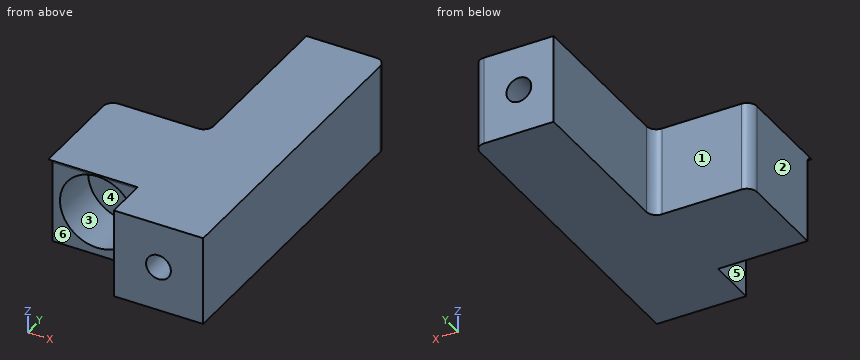
```python
from build123d import *

# Parameters (mm, degrees)
SKETCH1_W           = 9
SKETCH1_H           = 9
BOSS_EXTRUDE1_DEPTH = 15
SKETCH2_R           = 3.75
CUT_EXTRUDE1_DEPTH  = 5
SKETCH3_W           = 9
SKETCH3_H           = 9
BOSS_EXTRUDE2_DEPTH = 20
BOSS_EXTRUDE3_REACH = 25.859
SKETCH6_W           = 10
SKETCH6_H           = 9
CUT_EXTRUDE3_DEPTH  = 5
FILLET2_R           = 1
SKETCH7_W           = 8
SKETCH7_H           = 9
BOSS_EXTRUDE4_DEPTH = 12.5
SKETCH4_R           = 1.25
CUT_EXTRUDE2_DEPTH  = 36.478866949
FILLET3_R           = 1


with BuildPart() as part:
    # Sketch1 → Boss-Extrude1 (new body)
    with BuildSketch(Plane(origin=(0, 0, 0), x_dir=(1, 0, 0), z_dir=(0, 1, 0))):
        Rectangle(SKETCH1_W, SKETCH1_H)
    extrude(amount=BOSS_EXTRUDE1_DEPTH)

    # Sketch2 → Cut-Extrude1 (cut)
    with BuildSketch(Plane.XZ):
        with Locations(Location((0, 0, 0), (0, 0, 270))):
            Circle(SKETCH2_R)
    extrude(amount=-CUT_EXTRUDE1_DEPTH, mode=Mode.SUBTRACT)

    # Sketch3 → Boss-Extrude2 (add)
    with BuildSketch(Plane(origin=(0, 15, 0), x_dir=(1, 0, 0), z_dir=(0, 1, 0))):
        with Locations((9, 0)):
            Rectangle(SKETCH3_W, SKETCH3_H)
    extrude(amount=-BOSS_EXTRUDE2_DEPTH)

    # Boss-Extrude3: up to this face of the body (flat: up to its plane)
    boss_extrude3_end = Plane(part.part.faces().sort_by_distance((4.5, -2.5, 0))[0])
    # Sketch5 → Boss-Extrude3 (add, up to the picked face)
    with BuildSketch(Plane.ZY.offset(4.5), mode=Mode.PRIVATE) as boss_extrude3_sk1:
        with BuildLine():
            Line((4.5, -0.75), (4.5, 0))
            Line((4.5, 0), (3.75, 0))
            ThreePointArc((3.75, 0), (4.280330086, -0.219669914), (4.5, -0.75))
        make_face()
    boss_extrude3_tool1 = split(extrude(boss_extrude3_sk1.sketch, amount=-BOSS_EXTRUDE3_REACH, mode=Mode.PRIVATE), bisect_by=boss_extrude3_end, keep=Keep.BOTH, mode=Mode.PRIVATE)
    add(boss_extrude3_tool1.solids().sort_by(Axis((-4.5, -0.167526, 4.332474), (1, 0, 0)))[0])

    # Sketch6 → Cut-Extrude3 (cut)
    with BuildSketch(Plane(origin=(0, 15, 0), x_dir=(1, 0, 0), z_dir=(0, 1, 0))):
        with Locations((0.5, 0)):
            Rectangle(SKETCH6_W, SKETCH6_H)
    extrude(amount=-CUT_EXTRUDE3_DEPTH, mode=Mode.SUBTRACT)

    # Fillet2
    fillet2_edges = [part.edges().sort_by_distance(p)[0] for p in [
        (-4.5, 10, 0),
        (5.5, 10, 0),
    ]]
    fillet(fillet2_edges, radius=FILLET2_R)

    # Sketch7 → Boss-Extrude4 (add)
    with BuildSketch(Plane(origin=(0, 15, 0), x_dir=(1, 0, 0), z_dir=(0, 1, 0))):
        with Locations((9.5, 0)):
            Rectangle(SKETCH7_W, SKETCH7_H)
    extrude(amount=BOSS_EXTRUDE4_DEPTH)

    # Sketch4 → Cut-Extrude2 (cut, through all)
    with BuildSketch(Plane.XZ.offset(5)):
        with Locations(Location((9, 0, 0), (0, 0, 270))):
            Circle(SKETCH4_R)
    extrude(amount=-CUT_EXTRUDE2_DEPTH, mode=Mode.SUBTRACT)

    # Fillet3
    fillet3_edges = [part.edges().sort_by_distance(p)[0] for p in [
        (13.5, 27.5, 0),
    ]]
    fillet(fillet3_edges, radius=FILLET3_R)


solid = part.part
```
Work out the finished part from the listing and answer in its coordinate system (mm). Face numbers are marked on the shaded views. A direction names the side the tool comes from. Round coordinates to 2 decimals unless told otherwise and drop trailing zeros. Order: outer loops, then holes, each group sorted by start corner. A loop starts at its lowest first (then second) coordinate and runs counter-clockwise, first axis right, second up.
Q1. A cutting plane is placed at A-A, the plane x = 9. Determine the outline of the cut face in (y, z).
Solution:
outline: (-5, -4.5) - (27.5, -4.5) - (27.5, -1.25) - (-5, -1.25) - close; (-5, 1.25) - (27.5, 1.25) - (27.5, 4.5) - (-5, 4.5) - close
Q2. A cutting plane is placed at B-B, the plane z = 0. Determine the outline of the cut face in (x, y).
Solution:
outline: (-4.5, 0) - (-3.75, 0) - (-3.75, 5) - (3.75, 5) - (3.75, 0) - (4.5, 0) - (4.5, -5) - (7.75, -5) - (7.75, 27.5) - (5.5, 27.5) - (5.5, 11) arc R1 cw to (4.5, 10) - (-3.5, 10) arc R1 ccw to (-4.5, 9) - close; (10.25, -5) - (13.5, -5) - (13.5, 26.5) arc R1 ccw to (12.5, 27.5) - (10.25, 27.5) - close
Q3. Find the intervals of material crossed by line 1 along X through (y, z) = (1.5, 0); line 2 along X through (y, z) = (19, 0); line 3 along Y through (x, z) = (0, 3.5), in increasing order.
Solution:
line 1: x = -4.5 to -3.75, 3.75 to 7.75, 10.25 to 13.5
line 2: x = 5.5 to 7.75, 10.25 to 13.5
line 3: y = 5 to 10
Q4. Given pin 1 Ø4 at (x, z) = (-0.5, 1) entering from +Y; pin 2 Ø1.5 at (y, z) = (-2, -0.5) entering from -X; pin 3 Ø2 at (x, z) = (9, 0) entering from -Y, each flat-ended and moving along its own axis, determine where each tip first touches the part or whether it passes through.
Solution:
pin 1: stops at y = 10
pin 2: stops at x = 4.5
pin 3: passes through
Q5. A cutting plane is placed at D-D, the plane y = 20. Determine the outline of the cut face in (x, z), then the cut area to 3 significant figures.
Solution:
outline: (5.5, -4.5) - (13.5, -4.5) - (13.5, 4.5) - (5.5, 4.5) - close; hole circle Ø2.5 at (9, 0)
area: 67.1 mm2
Q6. A tool of negligible diameter and unlimited length cuts with its end or side. For the marked faces 1, 2 and 3, from which of +Z, -Z, +X, -X, +Y, -Y can it reach the whole face along a straight path? Write none if from no direction.
Solution:
face 1: +Z, -Z, -X, +Y
face 2: +Z, -Z, -X, +Y, -Y
face 3: -Y
Q7. A cutting plane is placed at C-C, the plane y = 6.5. Determine the outline of the cut face in (x, z).
Solution:
outline: (-4.5, -4.5) - (13.5, -4.5) - (13.5, 4.5) - (-4.5, 4.5) - close; hole circle Ø2.5 at (9, 0)
Q8. The mould has two halves that part along X. Classify the marked faces 4, 5 and 6: pulls with the +X half, pulls with the -X half, needs draft (parallel to the pull), parting line crosses it, or undercut.
Solution:
face 4: undercut
face 5: pulls with the -X half
face 6: needs draft
